Read the model definition and answer for the solid it produces. Units are mm, in the model's axes. A direction names the side the tool comes from. Coordinates: 2 decimals unless noted, no trailing zeros. Write each loop counter-clockwise with the first axis right and the second up, starting at its lowest first coordinate (ties: lowest second). Pieces come first, ordered by that corner, then holes. Notation, with made-up numbers: (77, -17.5) - (109, -17.5) arc R23 cw to (109, 16.5) - close; hole circle Ø1 at (8, 16.25). An arc over 180 degrees is marked (long way). Use a Markdown table: item, result.
from build123d import *

# Parameters (mm, degrees)
BOSS_EXTRUDE1_DEPTH = 128
CUT_EXTRUDE1_DEPTH  = 238.865508218
CUT_EXTRUDE2_START  = 50
CUT_EXTRUDE2_DEPTH  = 90
FILLET1_R           = 10


# Read off the part's stored shape, not the designer's step: Cut-Extrude2
with BuildPart() as part:
    # Sketch1 → Boss-Extrude1 (new body)
    with BuildSketch(Plane.XY):
        Polygon((0, 24), (26, 24), (26, 64), (164, 64), (164, 24), (190, 24), (190, 0), (0, 0), align=None)
    extrude(amount=-BOSS_EXTRUDE1_DEPTH)

    # Sketch5 → Cut-Extrude1 (cut, through all)
    with BuildSketch(Plane(origin=(0, 64, 0), x_dir=(1, 0, 0), z_dir=(0, 1, 0))):
        Polygon((0, 90), (26, 90), (50, 128), (0, 128), align=None)
        Polygon((164, 90), (190, 90), (190, 128), (140, 128), align=None)
    extrude(amount=-CUT_EXTRUDE1_DEPTH, mode=Mode.SUBTRACT)

    # Cut-Extrude2 outline → Cut-Extrude2 (cut)
    with BuildSketch(Plane.YZ.offset(CUT_EXTRUDE2_START)):
        Polygon((0, 0), (64, -103), (64, 0), align=None)
    extrude(amount=CUT_EXTRUDE2_DEPTH, mode=Mode.SUBTRACT)

    # Fillet1
    fillet1_edges = [part.edges().sort_by_distance(p)[0] for p in [
        (26, 24, -45),
        (0, 24, -45),
        (190, 24, -45),
        (164, 24, -45),
        (50, 32, -128),
        (140, 32, -128),
    ]]
    fillet(fillet1_edges, radius=FILLET1_R)


solid = part.part
(1) The mould has two halves that part along X. Classify faces 1 (the flat face through (177, 13, -90)), 2 (the flat face through (50, 46, -28)), 3 (the cylindrical face through (22.99, 26.85, -45.63)): pulls with the +X half, pulls with the -X half, needs draft (parallel to the pull), parting line crosses it, or undercut.
Report:
| item | result |
|---|---|
| face 1 | needs draft |
| face 2 | undercut |
| face 3 | pulls with the -X half |
(2) A cutting plane is placed at C-C, the plane y = 30. Write down the section's boundary in (x, z).
Report:
| item | result |
|---|---|
| outline | (25.17, -90) - (26, -90) - (47.06, -123.34) arc R10 ccw to (55.51, -128) - (134.49, -128) arc R10 ccw to (142.94, -123.34) - (164, -90) - (164.83, -90) - (164.83, 0) - (140, 0) - (140, -48.28) - (50, -48.28) - (50, 0) - (25.17, 0) - close |
(3) A cutting plane is placed at D-D, the plane x = 88.5. Write down the section's boundary in (y, z).
Report:
| item | result |
|---|---|
| outline | (0, -128) - (64, -128) - (64, -103) - (0, 0) - close |
(4) A cutting plane is placed at B-B, the plane x = 29. Write down the section's boundary in (y, z).
Report:
| item | result |
|---|---|
| outline | (0, -94.75) - (64, -94.75) - (64, 0) - (0, 0) - close |
(5) For faces 4 (the flat face through (140, 46, -28)), 5 (the flat face through (13, 24, -44)), 6 (the flat face through (13, 13, -90)), determine the directions among +Z, -Z, +X, -X, +Y, -Y from which every point of the face is accessible in a straight line to the end or side of a thin tool.
Report:
| item | result |
|---|---|
| face 4 | +Z, +Y |
| face 5 | +Z, -Z, -X, +Y |
| face 6 | -Z, -X, +Y, -Y |
(6) A cutting plane is placed at A-A, the plane y = 21.5. Write down the section's boundary in (x, z), and give its area (3 significant figures).
Report:
| item | result |
|---|---|
| outline | (3.39, -90) - (26, -90) - (47.06, -123.34) arc R10 ccw to (55.51, -128) - (134.49, -128) arc R10 ccw to (142.94, -123.34) - (164, -90) - (186.61, -90) - (186.61, 0) - (140, 0) - (140, -34.6) - (50, -34.6) - (50, 0) - (3.39, 0) - close |
| area | 17,700 mm² |
(7) Straight lines are drawn through the part: L1, parallel to X at y = 55, z = -71.5; L2, parallel to Y at x = 178, z = -30.5; L3, parallel to X at y = 40, z = -71. For each, find the intervals that lie inside material, in ascending order.
Report:
| item | result |
|---|---|
| L1 | x = 26 to 50, 140 to 164 |
| L2 | y = 0 to 24 |
| L3 | x = 26 to 164 |
(8) Each of these flat-tipped pins is pushed along its axis until it touches: P1, Ø5, axis at y = 40.5, z = -27, coming from the +X side; P2, Ø12, axis at x = 117, y = 54.5, coming from the +Z side; P3, Ø2, axis at y = 15.5, z = -99, coming from the -X side. Where does it stop, or does it pass through?
Report:
| item | result |
|---|---|
| P1 | stops at x = 164 |
| P2 | stops at z = -78.05 |
| P3 | stops at x = 31.05 |
